CAD build for the part. Positions are in the model's coordinates, mm. Round coordinates to 2 decimals unless told otherwise and drop trailing zeros. Loops run counter-clockwise (first coordinate to the right, second up) from the corner with the lowest first, then second, coordinate; pieces in that order, holes last. Notation, with made-up numbers: M -38,52 L -31,52 A17 cw -31,72 Z; hole C 77.25,60 d4. An arc over 180 degrees is marked long. Use a Markdown table: item, result. Add a question column.
(1) Flat gauge pins, fed straight in: P1, Ø2.5, axis at x = 52.17, y = 0, coming from the -Z side; P2, Ø3, axis at x = 78, z = -17, coming from the +Y side; P3, Ø0.6, axis at x = -26, y = 0, coming from the -Z side. Where does each tip first touch, or does it go through?
(2) Band-saw the part on B-B, the plane y = 8. Give the number of separate pieces and of enclosed holes in the cut face, and give its area (3 significant figures).
(3) Band-saw the part on A-A, the plane x = -5.5. Write the cut outline in (y, z).
(4) Band-saw the part on C-C, the plane x = 73.5. Write the cut outline in (y, z), and give its area (3 significant figures).
(5) Wall check: L1, parallel to X at y = 0, z = -15.75; L2, parallel to Y at x = 68, z = 8; L3, parallel to Y at x = 67, z = 9. Give the ranges that are in metal, low to high.
(6) Two-plate mould, pull along Y, no slides. Class faces 1 (the face through (-91.976, -1.647, 5.229)), 2 (the face through (-45.591, -0.217, -19.277)), 3 (the face through (76.761, -1.323, 10.074)), 4 (the face through (51.005, 0, 0)): released by +Y, released by -Y, zero draft, split by the parting line, or undercut.
from build123d import *

# Parameters (mm, degrees)
F2_R          = 1.905
F3_DEPTH      = 29.4065909418
F3_DEPTH_BACK = 29.4065909418
F4_R          = 10.16
F5_DEPTH      = 50.8
F6_R          = 0.9525
F7_DEPTH      = 38.1


with BuildPart() as f1:
    # F0 (on Front) → F1 (revolve)
    with BuildSketch(Plane.XZ):
        Polygon((-76.7316836545, 14.3540199185), (-101.3946243259, 0), (101.8053756741, 0), (101.8053756741, 19.05), (80.1327452064, 23.306587711), (35.6063488341, 29.4055909418), (-11.9658752189, 29.4055909418), (-56.4698129892, 23.1448132545), align=None)
    revolve(axis=Axis((0.2053756741, 0, 0), (1, 0, 0)))

    # F2 (on Front) → F3 (cut, two sides)
    with BuildSketch(Plane.XZ) as f3_sk:
        with Locations((-45.3427098691, -21.1661662906)):
            Circle(F2_R)
        with Locations((66.7973011732, -21.1661662906)):
            Circle(F2_R)
    extrude(amount=-F3_DEPTH, mode=Mode.SUBTRACT)
    extrude(f3_sk.sketch, amount=F3_DEPTH_BACK, mode=Mode.SUBTRACT)

    # F4 (on face) → F5 (cut)
    with BuildSketch(Plane.YZ.offset(101.8053756741)):
        Circle(F4_R)
    extrude(amount=-F5_DEPTH, mode=Mode.SUBTRACT)

    # F6 (on Top) → F7 (cut)
    with BuildSketch(Plane.XY):
        with Locations((-26.3292919844, 0)):
            Circle(F6_R)
        with Locations((52.1670617163, 0)):
            Circle(F6_R)
    extrude(amount=-F7_DEPTH, mode=Mode.SUBTRACT)


solid = f1.part
Return value:
| question | item | result |
|---|---|---|
| 1 | P1 | z = -27.31 |
| 1 | P2 | y = 17.82 |
| 1 | P3 | z = 0 |
| 2 | separate pieces | 1 |
| 2 | enclosed holes | 2 |
| 2 | area | 8,190 mm^2 |
| 3 | outline | C 0,0 d58.81 |
| 4 | outline | C 0,0 d48.43; hole C 0,0 d20.32 |
| 4 | area | 1,520 mm^2 |
| 5 | L1 | -73.51 to -27.28, -25.38 to 51.21, 53.12 to 101.81 |
| 5 | L2 | -23.65 to -6.26, 6.26 to 23.65 |
| 5 | L3 | -23.44 to -4.71, 4.71 to 23.44 |
| 6 | face 1 | split by the parting line |
| 6 | face 2 | zero draft |
| 6 | face 3 | undercut |
| 6 | face 4 | undercut |
